Read the model definition and answer for the solid it produces. Units are mm, in the model's axes. Round coordinates to 2 decimals unless told otherwise and drop trailing zeros. Order: outer loops, then holes, each group sorted by start corner. A loop starts at its lowest first (then second) coordinate and runs counter-clockwise, first axis right, second up. Notation, with made-up numbers: (75.25, 24.5) -> (92.25, 24.5) arc R7 cw to (92.25, 30.5) -> close; hole circle Ø5 at (-22, 3.25). An arc over 180 degrees is marked (long way). Answer as a JSON object with one key per item and string values. Group by question number.
Item 1: Section B-B, the plane z = 54.5 is taken. Write down the section's boundary in (x, y) (3 decimals).
Item 2: Consider probe 1 along Z at (x, y) = (-12.7, 1.55); probe 2 along Z at (x, y) = (107.24, 1.4); probe 3 along X at (y, z) = (1.6, 58.9). Determine where each line is inside the solid, lowest interval first. Write a range as from..to.
Item 3: Section A-A, the plane y = 1.6 is taken. Count the separate pieces of the cut face and the enclosed holes in it, plus the area to 3 significant figures.
from build123d import *

# Parameters (mm, degrees)
SKETCH1_R           = 1.63195
BOSS_EXTRUDE1_DEPTH = 3.175


with BuildPart() as part:
    # Sketch1 → Boss-Extrude1 (new body)
    with BuildSketch(Plane(origin=(0, 0, 0), x_dir=(1, 0, 0), z_dir=(0, 1, 0))):
        with BuildLine():
            Line((-66.2, 88.9), (97.24, 88.9))
            Line((97.24, 88.9), (142.24, 37.5))
            Line((142.24, 37.5), (142.24, -37.5))
            Line((142.24, -37.5), (97.24, -88.9))
            Line((97.24, -88.9), (-66.2, -88.9))
            ThreePointArc((-66.2, -88.9), (-73.271067812, -85.971067812), (-76.2, -78.9))
            Line((-76.2, -78.9), (-76.2, 78.9))
            ThreePointArc((-76.2, 78.9), (-73.271067812, 85.971067812), (-66.2, 88.9))
        make_face()
        with Locations((-12.7, 12.7)):
            Circle(SKETCH1_R, mode=Mode.SUBTRACT)
        with Locations((12.7, 12.7)):
            Circle(SKETCH1_R, mode=Mode.SUBTRACT)
        with Locations((12.7, -12.7)):
            Circle(SKETCH1_R, mode=Mode.SUBTRACT)
        with Locations((-12.7, -12.7)):
            Circle(SKETCH1_R, mode=Mode.SUBTRACT)
        with Locations((-50.8, 69.85)):
            Circle(SKETCH1_R, mode=Mode.SUBTRACT)
        with Locations((107.24, 58.9)):
            Circle(SKETCH1_R, mode=Mode.SUBTRACT)
        with Locations((107.24, -58.9)):
            Circle(SKETCH1_R, mode=Mode.SUBTRACT)
        with Locations((-50.8, -69.85)):
            Circle(SKETCH1_R, mode=Mode.SUBTRACT)
    extrude(amount=BOSS_EXTRUDE1_DEPTH)


solid = part.part
Values found:
{
 "1": {"outline": "(-76.2, 0) -> (127.357, 0) -> (127.357, 3.175) -> (-76.2, 3.175) -> close"},
 "2": {"probe 1": "-88.9..-14.33, -11.07..11.07, 14.33..88.9", "probe 2": "-77.48..-60.53, -57.27..57.27, 60.53..77.48", "probe 3": "-76.2..105.61, 108.87..123.5"},
 "3": {"separate pieces": "1", "enclosed holes": "8", "area": "36,400 mm2"}
}
